from build123d import *

# Parameters (mm, degrees)
BODY_DEPTH = 6.35


with BuildPart() as part:
    # Sketch1 → Body (new body)
    with BuildSketch(Plane(origin=(0, 0, 0), x_dir=(1, 0, 0), z_dir=(0, 1, 0))):
        Polygon((-49.076012748, 5.505075896), (-42.726012748, 5.505075896), (-42.726012748, 15.505075896), (27.273987252, 15.505075896), (27.273987252, 5.505075896), (33.623987252, 5.505075896), (33.623987252, -24.494924104), (27.273987252, -24.494924104), (27.273987252, -34.494924104), (-42.726012748, -34.494924104), (-42.726012748, -24.494924104), (-49.076012748, -24.494924104), align=None)
    extrude(amount=BODY_DEPTH)


solid = part.part
Model file for the job. Use its own axes, mm. A direction names the side the tool comes from. Round coordinates to 2 decimals unless told otherwise and drop trailing zeros. Loops run counter-clockwise (first coordinate to the right, second up) from the corner with the lowest first, then second, coordinate; pieces in that order, holes last. Notation, with made-up numbers: M 88,-9.5 L 107,-9.5 A14 ccw 107,-0.5 Z; hole C 38,-27 d6. An arc over 180 degrees is marked long. One line per question, with ' | ' between items.
1) Drill centre lines: line 1 along X through (y, z) = (2, 27); line 2 along Z through (x, y) = (-44.5, 0.5). Where is each one in solid material? Low to high.
Solved:
line 1: x = -42.73 to 27.27 | line 2: z = -5.51 to 24.49
2) Band-saw the part on B-B (z = -10). Give the cut face in (x, y).
Solved:
outline: M -42.73,0 L 27.27,0 L 27.27,6.35 L -42.73,6.35 Z
3) Band-saw the part on A-A (y = 2.75). Give the cut face in (x, z).
Solved:
outline: M -49.08,-5.51 L -42.73,-5.51 L -42.73,-15.51 L 27.27,-15.51 L 27.27,-5.51 L 33.62,-5.51 L 33.62,24.49 L 27.27,24.49 L 27.27,34.49 L -42.73,34.49 L -42.73,24.49 L -49.08,24.49 Z
4) Flat gauge pins, fed straight in: pin 1 (1.9 mm diameter, centred on x = 30.5, y = 3, fed in from +Z); pin 2 (1.9 mm diameter, centred on x = 29.5, y = 2, fed in from -Z); pin 3 (3 mm diameter, centred on y = 3, z = 27.5, fed in from -X). Where does each tip first touch, or does it go through?
Solved:
pin 1: stops at z = 24.49 | pin 2: stops at z = -5.51 | pin 3: stops at x = -42.73
5) 3-axis set-ups, long thin cutter, end or side, ignore diameter. For faces 1 (the flat face through (-46, 3, 24.495)), 2 (the flat face through (33.624, 3, 9)), 3 (the flat face through (30, 3, -5.505)), 4 (the flat face through (-46, 3, -5.505)), 5 (the flat face through (30, 3, 24.495)): which of +Z, -Z, +X, -X, +Y, -Y reach the whole face in a straight line?
Solved:
face 1: +Z, -X, +Y, -Y | face 2: +Z, -Z, +X, +Y, -Y | face 3: -Z, +X, +Y, -Y | face 4: -Z, -X, +Y, -Y | face 5: +Z, +X, +Y, -Y
